Can you work these out from the model? Positions are in its coordinate system, mm. Face numbers are marked on the shaded views. A direction names the side the tool comes from. Round coordinates to 2 decimals unless told otherwise and drop trailing zeros. Loops run counter-clockwise (first coordinate to the right, second up) from the corner with the lowest first, then second, coordinate; pieces in that order, holes last. Notation, with made-up numbers: M 40,-13 L 77,-13 A25 ccw 77,0 Z; hole C 37,-25.75 d7. An arc over 180 degrees is marked long. Return JSON: item names as keys, results as strings.
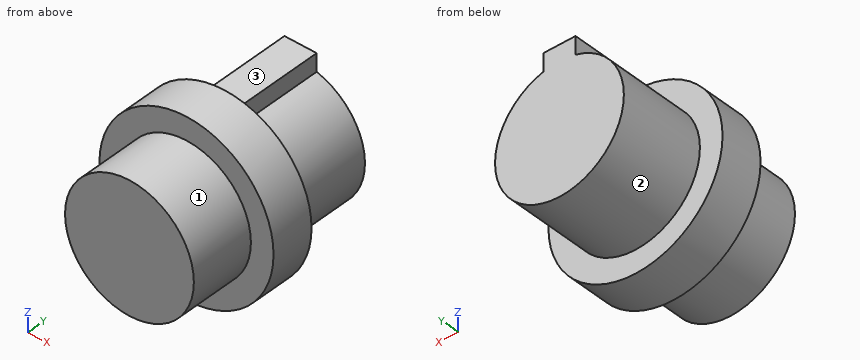
```python
from build123d import *

# Parameters (mm, degrees)
SKETCH1_R                = 9.398
BOSS_EXTRUDE1_DEPTH      = 9.525
SKETCH2_R                = 12.7
BOSS_EXTRUDE2_DEPTH      = 6.35
SKETCH3_R                = 9.398
BOSS_EXTRUDE3_DEPTH      = 12.7
BOSS_EXTRUDE4_REACH      = 41.654
BOSS_EXTRUDE4_END_RADIUS = 9.398
SKETCH4_W                = 4.699
SKETCH4_H                = 12.7


with BuildPart() as part:
    # Sketch1 → Boss-Extrude1 (new body)
    with BuildSketch(Plane(origin=(0, 0, 0), x_dir=(1, 0, 0), z_dir=(0, 1, 0))):
        with Locations(Location((0, 0, 0), (0, 0, 90))):
            Circle(SKETCH1_R)
    extrude(amount=BOSS_EXTRUDE1_DEPTH)

    # Sketch2 → Boss-Extrude2 (add)
    with BuildSketch(Plane(origin=(0, 9.525, 0), x_dir=(1, 0, 0), z_dir=(0, 1, 0))):
        with Locations(Location((0, 0, 0), (0, 0, 270))):
            Circle(SKETCH2_R)
    extrude(amount=BOSS_EXTRUDE2_DEPTH)

    # Sketch3 → Boss-Extrude3 (add)
    with BuildSketch(Plane(origin=(0, 15.875, 0), x_dir=(1, 0, 0), z_dir=(0, 1, 0))):
        with Locations(Location((0, 0, 0), (0, 0, 90))):
            Circle(SKETCH3_R)
    extrude(amount=BOSS_EXTRUDE3_DEPTH)

    # Boss-Extrude4: up to this cylinder (the profile starts outside it)
    boss_extrude4_end = Plane(origin=(0, 22.225, 0), z_dir=(0, -1, 0)) * Cylinder(BOSS_EXTRUDE4_END_RADIUS, 103.104, mode=Mode.PRIVATE)
    # Sketch4 → Boss-Extrude4 (add, up to the surface)
    with BuildSketch(Plane.XY.offset(11.684), mode=Mode.PRIVATE) as boss_extrude4_sk1:
        with Locations((0, 22.225)):
            Rectangle(SKETCH4_W, SKETCH4_H)
    boss_extrude4_tool1 = extrude(boss_extrude4_sk1.sketch, amount=-BOSS_EXTRUDE4_REACH, mode=Mode.PRIVATE) - boss_extrude4_end
    add(boss_extrude4_tool1.solids().sort_by_distance((0, 22.225, 11.684))[0])


solid = part.part
```
Q1. Suppose I cut it at C-C, the plane y = 19.5. Please give me the cut outline in (x, z).
Results:
{"outline": "M -2.35,9.1 A9.4 ccw long 2.35,9.1 L 2.35,11.68 L -2.35,11.68 Z"}
Q2. If I drill on line 1 along Y through (x, z) = (6, -8.25) (3 decimals); line 2 along X through (y, z) = (17, 10.5); line 3 along X through (y, z) = (23.5, 3.5), over which ranges is the centre line in solid material (lowest first)?
Results:
{"line 1": "y = 9.525 to 15.875", "line 2": "x = -2.35 to 2.35", "line 3": "x = -8.72 to 8.72"}
Q3. I'm going to push flat-ended pins straight in: pin 1 Ø1.5 at (x, y) = (-9.5, 9.5) entering from -Z; pin 2 Ø2 at (x, y) = (-4.5, 15) entering from +Z; pin 3 Ø1.4 at (x, y) = (0.5, 19.5) entering from +Z. Where does each tip first touch, or does it pass through?
Results:
{"pin 1": "stops at z = -9.2", "pin 2": "stops at z = 12.21", "pin 3": "stops at z = 11.68"}
Q4. On a 3-axis mill with a long thin cutter (end or side, diameter ignored), from which of +Z, -Z, +X, -X, +Y, -Y can I reach the whole of each face in a straight line? I mean the marked faces 1, 2 and 3. Say none if no direction works.
Results:
{"face 1": "-Y", "face 2": "+Y", "face 3": "+Z, +X, -X, +Y"}
Q5. Suppose I cut it at A-A, the plane x = 0. Please give me the cut outline in (y, z) (3 decimals).
Results:
{"outline": "M 0,-9.398 L 9.525,-9.398 L 9.525,-12.7 L 15.875,-12.7 L 15.875,-9.398 L 28.575,-9.398 L 28.575,11.684 L 15.875,11.684 L 15.875,12.7 L 9.525,12.7 L 9.525,9.398 L 0,9.398 Z"}
Q6. Suppose I cut it at D-D, the plane y = 12.5. Please give me the cut outline in (x, z).
Results:
{"outline": "C 0,0 d25.4"}
Q7. Suppose I cut it at B-B, the plane z = 0. Please give me the cut outline in (x, y) (3 decimals), plus the area to 3 significant figures.
Results:
{"outline": "M -12.7,9.525 L -9.398,9.525 L -9.398,0 L 9.398,0 L 9.398,9.525 L 12.7,9.525 L 12.7,15.875 L 9.398,15.875 L 9.398,28.575 L -9.398,28.575 L -9.398,15.875 L -12.7,15.875 Z", "area": "579 mm2"}
